Model file for the job. Use its own axes, mm. A direction names the side the tool comes from. Coordinates: 2 decimals unless noted, no trailing zeros. Order: outer loops, then holes, each group sorted by start corner. A loop starts at its lowest first (then second) coordinate and runs counter-clockwise, first axis right, second up. Notation, with made-up numbers: (89, 10) -> (123, 10) arc R24 ccw to (123, 23) -> close; hole circle Ø9 at (78, 47.5). An arc over 180 degrees is marked (long way). Return JSON: item names as keys, results as strings. Group by question number.
1) Cut at A-A (z = 11). Write the cut outline in (x, y).
2) Which spindle directions (+Z, -Z, +X, -X, +Y, -Y) get a long thin tool onto all of the face, cutting with end or side? Do faces 1 (the cylindrical face through (0, -5, 14)), 2 (the flat face through (9, 2.713, 12)), 3 (the cylindrical face through (8.3, -16.21, 2.46)). Say none if no direction does.
3) Flat gauge pins, fed straight in: pin 1 (2 mm diameter, centred on x = 0.5, y = 0, fed in from -Z); pin 2 (1.5 mm diameter, centred on x = 10, z = 15, fed in from +Y); pin 3 (6 mm diameter, centred on y = -9.5, z = 13.5, fed in from +X); pin 4 (1.6 mm diameter, centred on y = -0.5, z = 11, fed in from -X). Where does each tip first touch, or does it go through?
4) Probe line 1 (Y direction, x = 8.5, z = 2.2); line 2 (Y direction, x = -12, z = 6.75); line 3 (Y direction, x = -8, z = 17.75). List the from-to ranges inside material, lowest first.
5) Cut at B-B (x = 8.5). State how many separate pieces and enclosed holes the cut face has, and give its area (3 significant figures).
6) Pull direction X, two halves, no side cores. Call faces 4 (the flat face through (0, 2, 18)), 5 (the cylindrical face through (-9, 40, 9)), 6 (the cylindrical face through (-0.195, -18.487, 2.465)): +X half, -X half, draft (parallel to the pull), parting line (faces both ways), or undercut.
from build123d import *

# Parameters (mm, degrees)
F5_DEPTH  = 8
F6_DEPTH  = 9
F7_R      = 1.4
F8_DEPTH  = 54.201
F10_DEPTH = 18.001
F12_DEPTH = 26.4
F14_DEPTH = 18.001
F16_DEPTH = 5
F17_SIZE  = 0.5
F18_R     = 1.5
F19_DEPTH = 18.0010001


# Not quite as in the source:
# - a fillet or chamfer that OpenCascade refuses, or shapes differently, is made with other operations: its cross-section is extruded or revolved along the edge and cut away or added


with BuildPart() as f1:
    # F0 (on Front) → F1 (revolve)
    with BuildSketch(Plane.XZ):
        Polygon((0, 10), (0, 0), (41, 0), (41, 2), (40.5, 2), (40.5, 8), (41, 8), (41, 10), (30.5, 10), (30.5, 5), (5, 5), (5, 10), align=None)
    revolve(axis=Axis((0, 0, 5), (0, 0, -1)))

    # F2: fillet of radius 10 on 1 edges, made by hand

    # F2_s1 → F2_t2 (revolve)
    with BuildSketch(Plane.XZ):
        with BuildLine():
            ThreePointArc((13.6602540378, 5), (8.6602540378, 6.3397459622), (5, 10))
            Line((5, 10), (5, 5))
            Line((5, 5), (13.6602540378, 5))
        make_face()
    revolve(axis=Axis((0, 0, 5), (0, 0, -1)))

    # F3: fillet of radius 10 on 1 edges, made by hand

    # F3_s1 → F3_t2 (revolve)
    with BuildSketch(Plane.XZ):
        with BuildLine():
            ThreePointArc((30.5, 10), (26.8397459622, 6.3397459622), (21.8397459622, 5))
            Line((21.8397459622, 5), (30.5, 5))
            Line((30.5, 5), (30.5, 10))
        make_face()
    revolve(axis=Axis((0, 0, 5), (0, 0, -1)))

    # F4 (on face) → F5 (join)
    with BuildSketch(Plane.XY.offset(10)):
        with BuildLine():
            Line((-4.2, 2.7129319933), (-4.2, -2.7129319933))
            ThreePointArc((-4.2, -2.7129319933), (5, 0), (-4.2, 2.7129319933))
        make_face()
        Polygon((1.3, -0.7505553499), (0, -1.5011106999), (-1.3, -0.7505553499), (-1.3, 0.7505553499), (0, 1.5011106999), (1.3, 0.7505553499), align=None, mode=Mode.SUBTRACT)
    extrude(amount=F5_DEPTH)

    # F6 (add): a face of the model
    f6_faces = [f1.faces().sort_by_distance(p)[0] for p in [
        (-4.2, 0, 14),
    ]]
    extrude(f6_faces, amount=F6_DEPTH)

    # F7 (on face) → F8 (cut, through all)
    with BuildSketch(Plane(origin=(-13.2, 0, 0), x_dir=(0, -1, 0), z_dir=(-1, 0, 0))):
        with Locations((0, 14)):
            Circle(F7_R)
    extrude(amount=-F8_DEPTH, mode=Mode.SUBTRACT)

    # F9 (on face) → F10 (cut, through all)
    with BuildSketch(Plane.XY.offset(18)):
        Polygon((0, -1.5011106999), (1.3, -0.7505553499), (1.3, 0.7505553499), (0, 1.5011106999), (-1.3, 0.7505553499), (-1.3, -0.7505553499), align=None)
    extrude(amount=-F10_DEPTH, mode=Mode.SUBTRACT)

    # F11: fillet of radius 2 on 2 edges, made by hand

    # F11_s1 → F11_t2 (revolve)
    with BuildSketch(Plane.XZ):
        with BuildLine():
            ThreePointArc((40.5, 3.3228756555), (40.6291713066, 2.6157688743), (41, 2))
            Line((41, 2), (40.5, 2))
            Line((40.5, 2), (40.5, 3.3228756555))
        make_face()
    revolve(axis=Axis((0, 0, 2), (0, 0, -1)))

    # F11_s3 → F11_t4 (revolve)
    with BuildSketch(Plane.XZ):
        with BuildLine():
            ThreePointArc((41, 8), (40.6291713066, 7.3842311257), (40.5, 6.6771243445))
            Line((40.5, 6.6771243445), (40.5, 8))
            Line((40.5, 8), (41, 8))
        make_face()
    revolve(axis=Axis((0, 0, 8), (0, 0, -1)))

    # F12 (add): a face of the model
    f12_faces = [f1.faces().sort_by_distance(p)[0] for p in [
        (-13.2, 2.6162676255, 14),
    ]]
    extrude(f12_faces, amount=-F12_DEPTH)

    # F13 (on face) → F14 (cut, through all)
    with BuildSketch(Plane(origin=(0, 0, 0), x_dir=(1, 0, 0), z_dir=(0, 0, -1))):
        Polygon((0, -1.5011106999), (1.3, -0.7505553499), (1.3, 0.7505553499), (0, 1.5011106999), (-1.3, 0.7505553499), (-1.3, -0.7505553499), align=None)
    extrude(amount=-F14_DEPTH, mode=Mode.SUBTRACT)

    # F15 (on face) → F16 (join, through all)
    with BuildSketch(Plane.XY.offset(10)):
        with BuildLine():
            Line((13.2, -2.7129319933), (13.2, 2.7129319933))
            Line((13.2, 2.7129319933), (4.2, 2.7129319933))
            ThreePointArc((4.2, 2.7129319933), (0, 5), (-4.2, 2.7129319933))
            Line((-4.2, 2.7129319933), (-13.2, 2.7129319933))
            Line((-13.2, 2.7129319933), (-13.2, -2.7129319933))
            Line((-13.2, -2.7129319933), (-4.2, -2.7129319933))
            ThreePointArc((-4.2, -2.7129319933), (0, -5), (4.2, -2.7129319933))
            Line((4.2, -2.7129319933), (13.2, -2.7129319933))
        make_face()
    extrude(amount=-F16_DEPTH)

    # F17
    f17_edges = [f1.edges().sort_by_distance(p)[0] for p in [
        (-13.2, 1.4, 14),
        (13.2, 1.4, 14),
    ]]
    chamfer(f17_edges, length=F17_SIZE)

    # F18 (on face) → F19 (cut, through all)
    with BuildSketch(Plane(origin=(0, 0, 0), x_dir=(1, 0, 0), z_dir=(0, 0, -1))):
        with Locations((0, 17)):
            Circle(F18_R)
        with Locations((-8.5, 14.7224318643)):
            Circle(F18_R)
        with Locations((-14.7224318643, 8.5)):
            Circle(F18_R)
        with Locations((-17, 0)):
            Circle(F18_R)
        with Locations((-14.7224318643, -8.5)):
            Circle(F18_R)
        with Locations((-8.5, -14.7224318643)):
            Circle(F18_R)
        with Locations((0, -17)):
            Circle(F18_R)
        with Locations((8.5, -14.7224318643)):
            Circle(F18_R)
        with Locations((14.7224318643, -8.5)):
            Circle(F18_R)
        with Locations((17, 0)):
            Circle(F18_R)
        with Locations((14.7224318643, 8.5)):
            Circle(F18_R)
        with Locations((8.5, 14.7224318643)):
            Circle(F18_R)
    extrude(amount=-F19_DEPTH, mode=Mode.SUBTRACT)


solid = f1.part
Answers below:
{
 "1": {"outline": "(-13.2, -2.71) -> (-4.2, -2.71) arc R5 ccw to (4.2, -2.71) -> (13.2, -2.71) -> (13.2, 2.71) -> (4.2, 2.71) arc R5 ccw to (-4.2, 2.71) -> (-13.2, 2.71) -> close; hole (-1.3, -0.75) -> (0, -1.5) -> (1.3, -0.75) -> (1.3, 0.75) -> (0, 1.5) -> (-1.3, 0.75) -> close"},
 "2": {"face 1": "+Z, -Y", "face 2": "+Z", "face 3": "+Z, -Z"},
 "3": {"pin 1": "stops at z = 0", "pin 2": "stops at y = 2.71", "pin 3": "passes through", "pin 4": "stops at x = -13.2"},
 "4": {"line 1": "y = -39.95 to -16.22, -13.22 to 13.22, 16.22 to 39.95", "line 2": "y = -38.68 to -24.73, -2.71 to 2.71, 24.73 to 38.68", "line 3": "y = -2.71 to 2.71"},
 "5": {"separate pieces": "3", "enclosed holes": "1", "area": "572 mm^2"},
 "6": {"face 4": "draft", "face 5": "parting line", "face 6": "undercut"}
}
